Autodesk Inventor part; units mm, degrees
ref_plane "YZ Plane" through (0, 0, 0) normal (1, 0, 0) x (0, 1, 0)
ref_plane "XZ Plane" through (0, 0, 0) normal (0, 1, 0) x (-1, 0, 0)
ref_plane "XY Plane" through (0, 0, 0) normal (0, 0, 1) x (1, 0, 0)
sketch "Sketch1" plane through (0, 0, 0) normal (0, 0, 1) x (1, 0, 0)
  circle A0 centre (0, 0) radius 32
  dimension "d0" = 64
extrude "Extrusion1" add sketch "Sketch1" along normal blind 80
sketch "Sketch2" plane through (0, 0, 80) normal (0, 0, 1) x (1, 0, 0)
  line L0 (-14, 0) -> (14, 0) construction
  circle A0 centre (14, 0) radius 6.5
  circle A1 centre (-14, 0) radius 6.5
  point P0 (0, 0)
  point P1 (0, 0)
  dimension "d3" = 28
  dimension "d4" = 13
  dimension "d5" = 13
extrude "Extrusion2" add sketch "Sketch2" along normal blind 7.4
sketch "Sketch3" plane through (-14, 0, 87.4) normal (0, 0, 1) x (1, 0, 0)
  point P0 (14, 0)
  point P1 (0, 0)
  point P2 (28, 0)
  dimension "d8" = 28
  dimension "d9" = 14
hole "Hole1" at (-14, 0, 87.4) at (14, 0, 87.4) direction (0, 0, -1) diameter 4.134 depth 14.2 tip angle 118
properties part number "Capw"
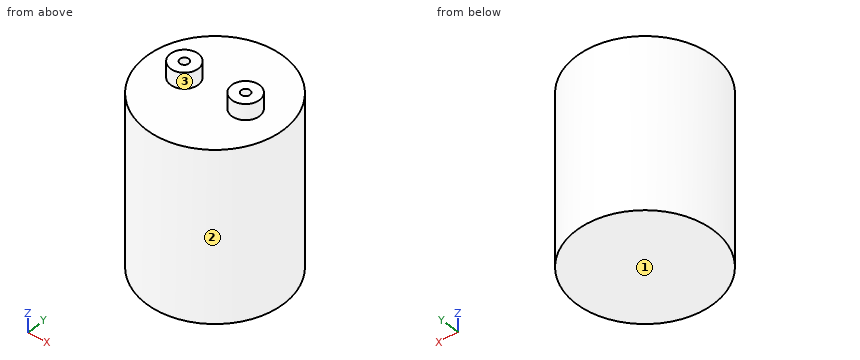
Build history of the part. All positions in model axes, mm. Face numbers are marked on the shaded views. Round coordinates to 2 decimals unless told otherwise and drop trailing zeros. Loops run counter-clockwise (first coordinate to the right, second up) from the corner with the lowest first, then second, coordinate; pieces in that order, holes last. Notation, with made-up numbers: (69, 50) -> (84, 50) arc R24 cw to (84, 84) -> close; hole circle Ø9 at (-20.75, -8). An arc over 180 degrees is marked (long way). Use CSV: the item, a comma, the result in double quotes. Start each with the question number.
Q1. Flat gauge pins, fed straight in: pin 1 Ø6 at (y, z) = (-25, 62.5) entering from -X; pin 2 Ø2 at (x, z) = (7, 46.5) entering from -Y; pin 3 Ø4 at (x, z) = (-12.5, 13) entering from +Y; pin 4 Ø19 at (x, y) = (-1, 9) entering from +Z. Where does each tip first touch, or does it go through?
Q2. Saw through at B-B on y = -5. Give the cut face in (x, z), and give its area (3 significant figures).
Q3. Saw through at D-D on x = -18. Give the cut face in (y, z).
Q4. Drill centre lines: L1, parallel to Y at x = -14, z = 83.5; L2, parallel to Z at x = 24.5, y = -4; L3, parallel to Y at x = 14, z = 76.75. Where is each one in solid material? Low to high.
Q5. Mould opens along X. For the marked faces 1, 2 and 3 say: +X half, -X half, draft (parallel to the pull), parting line (faces both ways), or undercut.
Q6. Saw through at C-C on z = 58. Give the cut face in (x, y).
Q7. Saw through at A-A on x = 0. Give the cut face in (y, z).
Solutions:
1,pin 1,"stops at x = -23.24"
1,pin 2,"stops at y = -31.43"
1,pin 3,"stops at y = 30.23"
1,pin 4,"stops at z = 87.4"
2,outline,"(-31.61, 0) -> (31.61, 0) -> (31.61, 80) -> (18.15, 80) -> (18.15, 87.4) -> (9.85, 87.4) -> (9.85, 80) -> (-9.85, 80) -> (-9.85, 87.4) -> (-18.15, 87.4) -> (-18.15, 80) -> (-31.61, 80) -> close"
2,area,"5,180 mm^2"
3,outline,"(-26.46, 0) -> (26.46, 0) -> (26.46, 80) -> (5.12, 80) -> (5.12, 87.4) -> (-5.12, 87.4) -> (-5.12, 80) -> (-26.46, 80) -> close"
4,L1,"y = -6.5 to -2.07, 2.07 to 6.5"
4,L2,"z = 0 to 80"
4,L3,"y = -28.77 to -2.07, 2.07 to 28.77"
5,face 1,"draft"
5,face 2,"parting line"
5,face 3,"undercut"
6,outline,"circle Ø64 at (0, 0)"
7,outline,"(-32, 0) -> (32, 0) -> (32, 80) -> (-32, 80) -> close"
